from build123d import *

# Parameters (mm, degrees)
BOSS_EXTRUDE1_DEPTH = 6
BOSS_EXTRUDE2_DEPTH = 2


with BuildPart() as part:
    # Sketch1 → Boss-Extrude1 (new body)
    with BuildSketch(Plane.XY):
        Polygon((-478.194997877, -284.039454162), (-470.194997877, -284.039454162), (-469.936178832, -284.005379989), (-469.694997877, -283.905479566), (-469.487891096, -283.746560944), (-469.328972474, -283.539454162), (-469.229072051, -283.298273207), (-469.194997877, -283.039454162), (-469.194997877, -277.439454162), (-425.194997877, -277.439454162), (-425.194997877, -283.039454162), (-425.160923704, -283.298273207), (-425.061023281, -283.539454162), (-424.902104659, -283.746560944), (-424.694997877, -283.905479566), (-424.453816922, -284.005379989), (-424.194997877, -284.039454162), (-416.194997877, -284.039454162), (-415.936178832, -284.005379989), (-415.694997877, -283.905479566), (-415.487891096, -283.746560944), (-415.328972474, -283.539454162), (-415.229072051, -283.298273207), (-415.194997877, -283.039454162), (-415.194997877, -277.439454162), (-407.194997877, -277.439454162), (-407.194997877, -272.439454162), (-461.194997877, -253.839454162), (-466.194997877, -253.839454162), (-466.194997877, -248.239454162), (-466.229072051, -247.980635117), (-466.328972474, -247.739454162), (-466.487891096, -247.532347381), (-466.694997877, -247.373428759), (-466.936178832, -247.273528336), (-467.194997877, -247.239454162), (-471.794997877, -247.239454162), (-472.053816922, -247.273528336), (-472.294997877, -247.373428759), (-472.502104659, -247.532347381), (-472.661023281, -247.739454162), (-472.760923704, -247.980635117), (-472.794997877, -248.239454162), (-472.794997877, -253.839454162), (-478.077534288, -253.839454162), (-478.077534288, -262.839454162), (-472.294997877, -262.839454162), (-472.294997877, -269.439454162), (-495.794997877, -269.439454162), (-495.794997877, -262.839454162), (-493.082722453, -262.839454162), (-493.082722453, -248.239454162), (-493.116796627, -247.980635117), (-493.21669705, -247.739454162), (-493.375615672, -247.532347381), (-493.582722453, -247.373428759), (-493.823903408, -247.273528336), (-494.082722453, -247.239454162), (-504.994997877, -247.239454162), (-505.253816922, -247.273528336), (-505.494997877, -247.373428759), (-505.702104659, -247.532347381), (-505.861023281, -247.739454162), (-505.960923704, -247.980635117), (-505.994997877, -248.239454162), (-505.994997877, -253.839454162), (-509.893267758, -253.839454162), (-509.893267758, -262.835675528), (-505.089806, -262.839454162), (-505.094997877, -269.439454162), (-509.893267758, -269.435677653), (-509.893267758, -277.439454162), (-504.694997877, -277.439454162), (-504.694997877, -283.039454162), (-504.660923704, -283.298273207), (-504.561023281, -283.539454162), (-504.402104659, -283.746560944), (-504.194997877, -283.905479566), (-503.953816922, -284.005379989), (-503.694997877, -284.039454162), (-495.694997877, -284.039454162), (-495.436178832, -284.005379989), (-495.194997877, -283.905479566), (-494.987891096, -283.746560944), (-494.828972474, -283.539454162), (-494.729072051, -283.298273207), (-494.694997877, -283.039454162), (-494.694997877, -277.439454162), (-479.194997877, -277.439454162), (-479.194997877, -283.039454162), (-479.160923704, -283.298273207), (-479.061023281, -283.539454162), (-478.902104659, -283.746560944), (-478.694997877, -283.905479566), (-478.453816922, -284.005379989), align=None)
        Polygon((-463.922205671, -257.066661956), (-463.636152151, -257.439454162), (-463.45633139, -257.873579881), (-463.394997877, -258.339454162), (-463.45633139, -258.805328444), (-463.636152151, -259.239454162), (-463.922205671, -259.612246369), (-464.294997877, -259.898299889), (-464.729123596, -260.07812065), (-465.194997877, -260.139454162), (-465.660872159, -260.07812065), (-466.094997877, -259.898299889), (-466.467790083, -259.612246369), (-466.753843604, -259.239454162), (-466.933664365, -258.805328444), (-466.994997877, -258.339454162), (-466.933664365, -257.873579881), (-466.753843604, -257.439454162), (-466.467790083, -257.066661956), (-466.094997877, -256.780608436), (-465.660872159, -256.600787675), (-465.194997877, -256.539454162), (-464.729123596, -256.600787675), (-464.294997877, -256.780608436), align=None, mode=Mode.SUBTRACT)
        Polygon((-503.1756105, -253.839454162), (-505.773686711, -258.339454162), (-503.1756105, -262.839454162), (-497.979458077, -262.839454162), (-495.381381866, -258.339454162), (-497.979458077, -253.839454162), align=None, mode=Mode.SUBTRACT)
    extrude(amount=-BOSS_EXTRUDE1_DEPTH)

    # Sketch1_4 → Boss-Extrude2 (add)
    with BuildSketch(Plane.XY):
        Polygon((-497.979458077, -262.839454162), (-495.381381866, -258.339454162), (-497.979458077, -253.839454162), (-503.1756105, -253.839454162), (-505.773686711, -258.339454162), (-503.1756105, -262.839454162), align=None)
        Polygon((-498.094928131, -254.039454162), (-503.060140446, -254.039454162), (-505.542746604, -258.339454162), (-503.060140446, -262.639454162), (-498.094928131, -262.639454162), (-495.612321973, -258.339454162), align=None, mode=Mode.SUBTRACT)
        Polygon((-495.612321973, -258.339454162), (-498.094928131, -254.039454162), (-503.060140446, -254.039454162), (-505.542746604, -258.339454162), (-503.060140446, -262.639454162), (-498.094928131, -262.639454162), align=None)
        Polygon((-498.210398185, -262.439454162), (-495.843262081, -258.339454162), (-498.210398185, -254.239454162), (-502.944670392, -254.239454162), (-505.311806496, -258.339454162), (-502.944670392, -262.439454162), align=None, mode=Mode.SUBTRACT)
        Polygon((-502.944670392, -262.439454162), (-498.210398185, -262.439454162), (-495.843262081, -258.339454162), (-498.210398185, -254.239454162), (-502.944670392, -254.239454162), (-505.311806496, -258.339454162), align=None)
        Polygon((-496.074202189, -258.339454162), (-498.325868239, -254.439454162), (-502.829200338, -254.439454162), (-505.080866388, -258.339454162), (-502.829200338, -262.239454162), (-498.325868239, -262.239454162), align=None, mode=Mode.SUBTRACT)
        Polygon((-498.325868239, -262.239454162), (-496.074202189, -258.339454162), (-498.325868239, -254.439454162), (-502.829200338, -254.439454162), (-505.080866388, -258.339454162), (-502.829200338, -262.239454162), align=None)
        Polygon((-496.305142296, -258.339454162), (-498.441338292, -254.639454162), (-502.713730284, -254.639454162), (-504.84992628, -258.339454162), (-502.713730284, -262.039454162), (-498.441338292, -262.039454162), align=None, mode=Mode.SUBTRACT)
        Polygon((-498.441338292, -262.039454162), (-496.305142296, -258.339454162), (-498.441338292, -254.639454162), (-502.713730284, -254.639454162), (-504.84992628, -258.339454162), (-502.713730284, -262.039454162), align=None)
        Polygon((-504.618986173, -258.339454162), (-502.598260231, -261.839454162), (-498.556808346, -261.839454162), (-496.536082404, -258.339454162), (-498.556808346, -254.839454162), (-502.598260231, -254.839454162), align=None, mode=Mode.SUBTRACT)
        Polygon((-502.598260231, -254.839454162), (-504.618986173, -258.339454162), (-502.598260231, -261.839454162), (-498.556808346, -261.839454162), (-496.536082404, -258.339454162), (-498.556808346, -254.839454162), align=None)
        Polygon((-502.482790177, -261.639454162), (-498.6722784, -261.639454162), (-496.767022512, -258.339454162), (-498.6722784, -255.039454162), (-502.482790177, -255.039454162), (-504.388046065, -258.339454162), align=None, mode=Mode.SUBTRACT)
        Polygon((-504.388046065, -258.339454162), (-502.482790177, -261.639454162), (-498.6722784, -261.639454162), (-496.767022512, -258.339454162), (-498.6722784, -255.039454162), (-502.482790177, -255.039454162), align=None)
        Polygon((-504.157105957, -258.339454162), (-502.367320123, -261.439454162), (-498.787748454, -261.439454162), (-496.99796262, -258.339454162), (-498.787748454, -255.239454162), (-502.367320123, -255.239454162), align=None, mode=Mode.SUBTRACT)
        Polygon((-502.367320123, -255.239454162), (-504.157105957, -258.339454162), (-502.367320123, -261.439454162), (-498.787748454, -261.439454162), (-496.99796262, -258.339454162), (-498.787748454, -255.239454162), align=None)
        Polygon((-503.475311767, -257.562997027), (-503.577534288, -258.339454162), (-503.475311767, -259.115911298), (-503.1756105, -259.839454162), (-502.698854632, -260.460774506), (-502.077534288, -260.937530374), (-501.353991424, -261.237231641), (-500.577534288, -261.339454162), (-499.801077153, -261.237231641), (-499.077534288, -260.937530374), (-498.456213945, -260.460774506), (-497.979458077, -259.839454162), (-497.67975681, -259.115911298), (-497.577534288, -258.339454162), (-497.67975681, -257.562997027), (-497.979458077, -256.839454162), (-498.456213945, -256.218133819), (-499.077534288, -255.741377951), (-499.801077153, -255.441676684), (-500.577534288, -255.339454162), (-501.353991424, -255.441676684), (-502.077534288, -255.741377951), (-502.698854632, -256.218133819), (-503.1756105, -256.839454162), align=None, mode=Mode.SUBTRACT)
    extrude(amount=-BOSS_EXTRUDE2_DEPTH)


solid = part.part
The listing builds one solid part. Answer for the finished solid, in the listing's coordinates (mm). A direction names the side the tool comes from. Coordinates: 2 decimals unless noted, no trailing zeros. Order: outer loops, then holes, each group sorted by start corner. A loop starts at its lowest first (then second) coordinate and runs counter-clockwise, first axis right, second up.
Q1. A cutting plane is placed at B-B, the plane z = -3.2. State how many separate pieces and enclosed holes the cut face has, and give its area (3 significant figures).
Q2. A cutting plane is placed at A-A, the plane y = -249.5. Write down the section's boundary in (x, z) (3 decimals), and give its area (3 significant figures).
Q3. Which of the six approach directions +Z, -Z, +X, -X, +Y, -Y give full straight-line access (tool end or side, diameter ignored) to faces 1 (the face through (-494, -262.839, -3)), 2 (the face through (-504.456, -256.058, -3.972)), 3 (the face through (-504.695, -280, -3)), 4 (the face through (-425.195, -280, -3)), 5 (the face through (-478.078, -258, -3))?
Q4. Given P1, Ø1.2, axis at x = -508.5, z = -3.5, coming from the +Y side; P2, Ø3, axis at x = -438.5, y = -275, coming from the +Z side; P3, Ø1.7, axis at y = -279.5, z = -2.5, coming from the -X side (3 decimals); P4, Ø3, axis at y = -280, z = -4.5, coming from the +X side (3 decimals), each flat-ended and moving along its own axis, determine where each tip first touches the part or whether it passes through.
Q5. For a pull along Y with two mould halves and no side action, classify faces 6 (the face through (-496.662, -256.121, -3.972)), 7 (the face through (-411, -277.439, -3)), 8 (the face through (-475, -253.839, -3)) as pulls with the +Y half, pulls with the -Y half, needs draft (parallel to the pull), parting line crosses it, or undercut.
Q6. Consider line 1 (X direction, y = -280.5, z = -1.75) (3 decimals); line 2 (Y direction, x = -494.5, z = -0.75); line 3 (Y direction, x = -467.5, z = -4.35). Determine where each line is inside the solid, lowest interval first.
Q7. A cutting plane is placed at C-C, the plane x = -491. Write down the section's boundary in (y, z), and give its area (3 significant figures).
Q8. A cutting plane is placed at D-D, the plane y = -268. Write down the section's boundary in (x, z) (3 decimals), and give its area (3 significant figures).
Answers follow:
1. separate pieces: 1
1. enclosed holes: 2
1. area: 1,840 mm2
2. outline: (-505.995, -6) - (-493.083, -6) - (-493.083, 0) - (-505.995, 0) - close; (-472.795, -6) - (-466.195, -6) - (-466.195, 0) - (-472.795, 0) - close
2. area: 117 mm2
3. face 1: +Z, -Z
3. face 2: -Z
3. face 3: +Z, -Z, -X, -Y
3. face 4: +Z, -Z, -Y
3. face 5: +Z, -Z, +Y
4. P1: stops at y = -253.84
4. P2: stops at z = 0
4. P3: stops at x = -504.695
4. P4: stops at x = -415.195
5. face 6: undercut
5. face 7: pulls with the -Y half
5. face 8: pulls with the +Y half
6. line 1: x = -504.695 to -494.695, -479.195 to -469.195, -425.195 to -415.195
6. line 2: y = -277.44 to -269.44, -262.84 to -247.24
6. line 3: y = -277.44 to -247.24
7. outline: (-277.44, -6) - (-269.44, -6) - (-269.44, 0) - (-277.44, 0) - close
7. area: 48.0 mm2
8. outline: (-505.094, -6) - (-495.795, -6) - (-495.795, 0) - (-505.094, 0) - close; (-472.295, -6) - (-420.084, -6) - (-420.084, 0) - (-472.295, 0) - close
8. area: 369 mm2
